Geometry: final body of the model. Coordinates: model frame, mm. Face numbers are marked on the shaded views. Give positions to 0.01 mm unless a question says otherwise; leave off trailing zeros. Order: outer loops, then holes, each group sorted by start corner. A loop starts at its lowest first (then second) coordinate and runs counter-clockwise, first axis right, second up. Notation, with made-up numbers: (67.5, -2) - (120.5, -2) arc R24 ccw to (120.5, 36) - close; hole circle Ø9 at (10, -10). An arc over 180 degrees is marked (long way). Use one line per item in the form item = value.
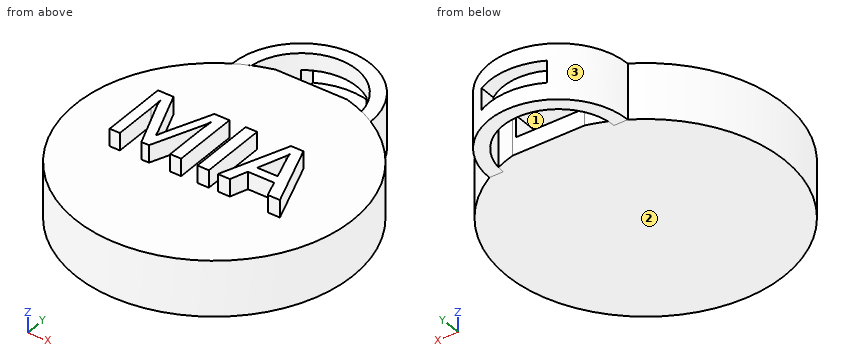
Autodesk Inventor part; units mm, degrees
ref_plane "YZ Plane" through (0, 0, 0) normal (1, 0, 0) x (0, 1, 0)
ref_plane "XZ Plane" through (0, 0, 0) normal (0, 1, 0) x (-1, 0, 0)
ref_plane "XY Plane" through (0, 0, 0) normal (0, 0, 1) x (1, 0, 0)
sketch "Sketch1" plane through (0, 0, 0) normal (0, 0, 1) x (1, 0, 0)
  circle A0 centre (0, 0) radius 12.7
  arc A1 (3.287, 12.2673) -> (-3.287, 12.2673) centre (0, 0) ccw
  line L0 (0, 0) -> (3.287, 12.2673) construction
  line L1 (0, 0) -> (12.7, 0) construction
  line L2 (0, 0) -> (-3.287, 12.2673) construction
  line L3 (-3.287, 12.2673) -> (3.287, 12.2673)
  point P0 (3.287, 12.2673)
  point P1 (-3.287, 12.2673)
  dimension "d0" = 25.4
  dimension "d1" = 12.7
  dimension "d2" = 75
  dimension "d3" = 30
extrude "Extrusion1" add sketch "Sketch1" along normal blind 5.08 contours A0 L3 picked at (4.079, -0.9801)
sketch "Sketch3" plane through (0, 0, 5.08) normal (0, 0, 1) x (1, 0, 0)
  arc A0 (-3.287, 12.2673) -> (3.287, 12.2673) centre (0, 0) ccw
  arc A1 (6.35, 10.9985) -> (-6.35, 10.9985) centre (0, 0) ccw
  line L0 (0, 0) -> (6.35, 10.9985) construction
  line L1 (0, 0) -> (12.7, 0) construction
  line L2 (0, 0) -> (-6.35, 10.9985) construction
  line L3 (-6.35, 10.9985) -> (6.35, 10.9985)
  dimension "d12" = 60
  dimension "d13" = 60
ref_plane "Work Plane1" through (-6.35, 10.9985, 5.08) normal (0, 1, 0) x (1, 0, 0)
sketch "Sketch4" plane through (-6.35, 10.9985, 5.08) normal (0, 1, 0) x (1, 0, 0)
  line L0 (-6.35, 0) -> (19.05, 0)
  line L1 (-6.35, 5.08) -> (19.05, 5.08)
  line L2 (-0.0044, 0) -> (12.6956, 0)
  line L3 (12.6956, 0) -> (12.6956, 5.08)
  line L4 (12.6956, 5.08) -> (-0.0044, 5.08)
  line L5 (-0.0044, 5.08) -> (-0.0044, 0)
  line L6 (-0.0044, 5.08) -> (1.2656, 5.08)
  line L7 (1.2656, 5.08) -> (1.2656, 0)
  line L8 (1.2656, 0) -> (-0.0044, 0)
  line L9 (-0.0044, 0) -> (-0.0044, 5.08)
  line L10 (12.6956, 0) -> (11.4256, 0)
  line L11 (11.4256, 0) -> (11.4256, 5.08)
  line L12 (11.4256, 5.08) -> (12.6956, 5.08)
  line L13 (12.6956, 5.08) -> (12.6956, 0)
  line L14 (6.35, 5.08) -> (6.3456, 0)
  point P0 (3.063, 0)
  point P1 (9.637, 0)
  point P2 (3.063, 5.08)
  point P3 (9.637, 5.08)
  dimension "d15" = 12.7
  dimension "d16" = 1.27
  dimension "d17" = 1.27
revolve "Revolution1" add sketch "Sketch4" angle 180 about axis through (0, 10.9985, 0) along (-0.0009, 0, 1) contours L11 L1 L3 L0
sketch "Sketch5" plane through (0, 0, 5.08) normal (0, 0, 1) x (1, 0, 0)
  line L0 (6.35, -3.175) -> (-6.35, -3.175)
  line L1 (-6.35, -3.175) -> (-6.35, 3.175)
  line L2 (-6.35, 3.175) -> (6.35, 3.175)
  line L3 (6.35, 3.175) -> (6.35, -3.175)
  line L4 (6.35, -3.175) -> (-6.35, 3.175) construction
  line L5 (-6.35, -3.175) -> (6.35, 3.175) construction
  line L6 (-9.525, 3.175) -> (9.525, 3.175) construction
  line L7 (9.525, 3.175) -> (9.525, -3.0049) construction
  line L8 (9.525, -3.0049) -> (-9.525, -3.0049) construction
  line L9 (-9.525, -3.0049) -> (-9.525, 3.175) construction
  line L10 (-6.35, 3.175) -> (-9.525, 3.175)
  line L11 (-0.9161, -2.921) -> (-1.917, -2.921)
  line L12 (-1.917, -2.921) -> (-1.917, 1.0261)
  spline S0 degree 2 poles (-1.917, 1.0261) (-1.917, 1.5125) (-1.8605, 2.2137) knots 0 0 0 1 1 1
  line L13 (-1.8605, 2.2137) -> (-1.8774, 2.2137)
  spline S1 degree 2 poles (-1.8774, 2.2137) (-1.9679, 1.8122) (-2.0414, 1.6369) knots 0 0 0 1 1 1
  line L14 (-2.0414, 1.6369) -> (-3.8623, -2.921)
  line L15 (-3.8623, -2.921) -> (-4.5579, -2.921)
  line L16 (-4.5579, -2.921) -> (-6.3844, 1.6029)
  spline S2 degree 2 poles (-6.3844, 1.6029) (-6.4579, 1.8009) (-6.5427, 2.2137) knots 0 0 0 1 1 1
  line L17 (-6.5427, 2.2137) -> (-6.5597, 2.2137)
  spline S3 degree 2 poles (-6.5597, 2.2137) (-6.5258, 1.8461) (-6.5258, 1.0148) knots 0 0 0 1 1 1
  line L18 (-6.5258, 1.0148) -> (-6.5258, -2.921)
  line L19 (-6.5258, -2.921) -> (-7.4645, -2.921)
  line L20 (-7.4645, -2.921) -> (-7.4645, 3.175)
  line L21 (-7.4645, 3.175) -> (-6.0395, 3.175)
  line L22 (-6.0395, 3.175) -> (-4.4391, -0.8852)
  spline S4 degree 2 poles (-4.4391, -0.8852) (-4.2525, -1.3546) (-4.1959, -1.5808) knots 0 0 0 1 1 1
  line L23 (-4.1959, -1.5808) -> (-4.179, -1.5808)
  spline S5 degree 2 poles (-4.179, -1.5808) (-4.0206, -1.1001) (-3.9245, -0.8683) knots 0 0 0 1 1 1
  line L24 (-3.9245, -0.8683) -> (-2.2902, 3.175)
  line L25 (-2.2902, 3.175) -> (-0.9161, 3.175)
  line L26 (-0.9161, 3.175) -> (-0.9161, -2.921)
  line L27 (1.623, -2.921) -> (0.5768, -2.921)
  line L28 (0.5768, -2.921) -> (0.5768, 3.175)
  line L29 (0.5768, 3.175) -> (1.623, 3.175)
  line L30 (1.623, 3.175) -> (1.623, -2.921)
  line L31 (8.1318, -2.921) -> (7.0234, -2.921)
  line L32 (7.0234, -2.921) -> (6.4749, -1.3716)
  line L33 (6.4749, -1.3716) -> (4.0772, -1.3716)
  line L34 (4.0772, -1.3716) -> (3.5456, -2.921)
  line L35 (3.5456, -2.921) -> (2.4429, -2.921)
  line L36 (2.4429, -2.921) -> (4.7275, 3.175)
  line L37 (4.7275, 3.175) -> (5.8641, 3.175)
  line L38 (5.8641, 3.175) -> (8.1318, -2.921)
  line L39 (6.2034, -0.5459) -> (5.3609, 1.8857)
  spline S6 degree 2 poles (5.3609, 1.8857) (5.3213, 2.0101) (5.276, 2.2702) knots 0 0 0 1 1 1
  line L40 (5.276, 2.2702) -> (5.2591, 2.2702)
  spline S7 degree 2 poles (5.2591, 2.2702) (5.2251, 2.0271) (5.1742, 1.8857) knots 0 0 0 1 1 1
  line L41 (5.1742, 1.8857) -> (4.3373, -0.5459)
  line L42 (4.3373, -0.5459) -> (6.2034, -0.5459)
  point P0 (0, 0)
  dimension "d19" = 12.7
  dimension "d20" = 6.35
  dimension "d21" = 19.05
  dimension "d22" = 3.175
extrude "Extrusion3" add sketch "Sketch5" along normal blind 1.5875 contours L33 L34 L35 L36 L2 L38 L3 | L3 L38 L31 L32 L33 | L16 S2 L17 S3 L18 L19 L20 L10 L1 | L1 L2 L22 S4 L23 S5 L24 L26 L11 L12 S0 L13 S1 L14 L15 L16 | L30 L27 L28 L2
sketch "Sketch2" plane through (-3.287, 12.2673, 0) normal (0, 1, 0) x (1, 0, 0)
  line L0 (6.574, 0) -> (0, 0)
  line L1 (6.574, -5.08) -> (0, -5.08)
  line L2 (0, 0) -> (6.574, 0)
  line L3 (6.574, 0) -> (6.574, -5.08)
  line L4 (6.574, -5.08) -> (0, -5.08)
  line L5 (0, -5.08) -> (0, 0)
  line L6 (3.287, 0) -> (3.287, -5.08)
  line L7 (0.287, -1.54) -> (6.287, -1.54)
  line L8 (6.287, -1.54) -> (6.287, -3.54)
  line L9 (6.287, -3.54) -> (0.287, -3.54)
  line L10 (0.287, -3.54) -> (0.287, -1.54)
  line L11 (0.287, -1.54) -> (6.287, -3.54) construction
  line L12 (6.287, -1.54) -> (0.287, -3.54) construction
  point P0 (3.287, -2.54)
  dimension "d6" = 6.574
  dimension "d8" = 6
  dimension "d9" = 2
extrude "Extrusion2" cut sketch "Sketch2" along normal blind 12.7 and the other way blind 17 contours L7 L8 L9 L6 | L6 L9 L10 L7
properties part number "MIA Pendant 2"
(1) Contact query for flat-ended pins moving along their axis: pin 1 Ø0.6 at (x, z) = (3, 6) entering from -Y; pin 2 Ø1.5 at (x, z) = (-8.5, 5.5) entering from -Y; pin 3 Ø2 at (x, y) = (0.5, -5.5) entering from -Z. Output: stop coordinate, or through.
Computed values:
pin_1 = -2.92
pin_2 = -9.96
pin_3 = 0
(2) Cut plane B-B on y = 6.5. Output: boundary loops of the cut face in (x, z), plus the area to 3 significant figures.
Computed values:
outline = (-10.91, 0) - (10.91, 0) - (10.91, 5.08) - (-10.91, 5.08) - close; hole (-3, 1.54) - (3, 1.54) - (3, 3.54) - (-3, 3.54) - close
area = 98.9 mm²
(3) Pull-direction query (X, two-part tool) for the marked faces 1, 2 and 3; classes: released by +X, released by -X, zero draft, split by the parting line, or undercut.
Computed values:
face_1 = undercut
face_2 = zero draft
face_3 = split by the parting line
(4) Ray query, line 1 along Z through (x, y) = (-2.75, 11.5); line 2 along Z through (x, y) = (-2.25, 2.5); line 3 along Z through (x, y) = (-3.5, 10). Return the intervals inside material, ascending.
Computed values:
line_1 = 0 to 1.54, 3.54 to 5.08
line_2 = 0 to 1.54, 3.54 to 6.67
line_3 = 0 to 5.08
(5) Cut plane A-A on z = 6. Give the number of separate pieces and of enclosed holes in the cut face, plus the area to 3 significant figures.
Computed values:
separate_pieces = 3
enclosed_holes = 1
area = 41.6 mm²
(6) Cut plane D-D on x = 8.5. Output: boundary loops of the cut face in (y, z).
Computed values:
outline = (-9.44, 0) - (9.44, 0) - (9.44, 5.08) - (-9.44, 5.08) - close
